Geometry check sheet. Reference: the model listing, model coordinates, mm. A direction names the side the tool comes from. Give positions to 0.01 mm unless a question says otherwise; leave off trailing zeros. Loops run counter-clockwise (first coordinate to the right, second up) from the corner with the lowest first, then second, coordinate; pieces in that order, holes last. Notation, with made-up numbers: (53, -40) -> (100, -40) arc R12 ccw to (100, -36) -> close; hole circle Ø10 at (22.5, 65). An arc over 180 degrees is marked (long way). Write item = value, one per line. Start each with the question number.
```python
from build123d import *

# Parameters (mm, degrees)
F0_W     = 600
F0_H     = 600
F1_DEPTH = 50
F2_W     = 600
F2_H     = 30
F3_DEPTH = 800
F5_DEPTH = 600


with BuildPart() as f1:
    # F0 (on Top) → F1 (new body)
    with BuildSketch(Plane.XY):
        Rectangle(F0_W, F0_H)
    extrude(amount=F1_DEPTH)

    # F2 (on face) → F3 (join)
    with BuildSketch(Plane.XY.offset(50)):
        with Locations((0, -285)):
            Rectangle(F2_W, F2_H)
    extrude(amount=F3_DEPTH)

    # F4 (on face) → F5 (join)
    with BuildSketch(Plane(origin=(0, 0, 0), x_dir=(1, 0, 0), z_dir=(0, 0, -1))):
        with BuildLine():
            Line((-250, 250), (-200, 250))
            ThreePointArc((-200, 250), (-214.644661, 285.355339), (-250, 300))
            ThreePointArc((-250, 300), (-285.355339, 285.355339), (-300, 250))
            ThreePointArc((-300, 250), (-285.355339, 214.644661), (-250, 200))
            Line((-250, 200), (-250, 250))
        make_face()
        with BuildLine():
            ThreePointArc((-250, 200), (-214.644661, 214.644661), (-200, 250))
            Line((-200, 250), (-250, 250))
            Line((-250, 250), (-250, 200))
        make_face()
        with BuildLine():
            ThreePointArc((250, 300), (214.644661, 285.355339), (200, 250))
            Line((200, 250), (250, 250))
            Line((250, 250), (250, 200))
            ThreePointArc((250, 200), (285.355339, 214.644661), (300, 250))
            ThreePointArc((300, 250), (285.355339, 285.355339), (250, 300))
        make_face()
        with BuildLine():
            ThreePointArc((-200, -250), (-214.644661, -214.644661), (-250, -200))
            Line((-250, -200), (-250, -250))
            Line((-250, -250), (-200, -250))
        make_face()
        with BuildLine():
            Line((-250, -250), (-250, -200))
            ThreePointArc((-250, -200), (-285.355339, -214.644661), (-300, -250))
            ThreePointArc((-300, -250), (-285.355339, -285.355339), (-250, -300))
            ThreePointArc((-250, -300), (-214.644661, -285.355339), (-200, -250))
            Line((-200, -250), (-250, -250))
        make_face()
        with BuildLine():
            Line((250, -250), (250, -200))
            ThreePointArc((250, -200), (214.644661, -214.644661), (200, -250))
            Line((200, -250), (250, -250))
        make_face()
        with BuildLine():
            ThreePointArc((300, -250), (285.355339, -214.644661), (250, -200))
            Line((250, -200), (250, -250))
            Line((250, -250), (200, -250))
            ThreePointArc((200, -250), (214.644661, -285.355339), (250, -300))
            ThreePointArc((250, -300), (285.355339, -285.355339), (300, -250))
        make_face()
        with BuildLine():
            Line((250, 250), (200, 250))
            ThreePointArc((200, 250), (214.644661, 214.644661), (250, 200))
            Line((250, 200), (250, 250))
        make_face()
    extrude(amount=F5_DEPTH)


solid = f1.part
```
1) Section check D-D (z = 762.5). Enter the section's corners in (x, y).
2) Draft check along X on faces 4 (the flat face through (290, -290, 0)), 5 (the flat face through (300, -90, 45)), 6 (the flat face through (-4, 4, 0)). Enter one of: released by +X, released by -X, zero draft, split by the parting line, or undercut.
3) Depth check by flat-ended pin: pin 1 Ø8 at (x, y) = (60.5, -204) entering from +Z. Enter the tip coordinate at first touch or a pass-through.
4) Section check A-A (z = -100.5). Enter the section's corners in (x, y), plus the area to 3 significant figures.
5) Section check B-B (x = 56). Enter the section's corners in (y, z), plus the area to 3 significant figures.
6) Tool access check on faces 1 (the flat face through (-290, 288, 0)), 2 (the flat face through (-290, -288, 0)), 3 (the flat face through (-4, -270, 444)). Record the directions out of +Z, -Z, +X, -X, +Y, -Y that give a thin tool (end or side, any length) a straight path to the whole face; none if there is none.
7) Thickness scan on line 1 (Z direction, x = 97, y = -217); line 2 (Z direction, x = -224, y = -217); line 3 (Y direction, x = -244, z = 522). Record the ranges inside material, lowest first.
8) Section check C-C (y = 215.5). Enter the section's corners in (x, z).
Check result:
q1.outline = (-300, -300) -> (300, -300) -> (300, -270) -> (-300, -270) -> close
q2.face_4 = zero draft
q2.face_5 = released by +X
q2.face_6 = undercut
q3.pin_1 = 50
q4.outline = circle Ø100 at (-250, -250); circle Ø100 at (-250, 250); circle Ø100 at (250, -250); circle Ø100 at (250, 250)
q4.area = 31,400 mm2
q5.outline = (-300, 0) -> (300, 0) -> (300, 50) -> (-270, 50) -> (-270, 850) -> (-300, 850) -> close
q5.area = 54,000 mm2
q6.face_1 = -Z, -X, +Y
q6.face_2 = -Z, -X, -Y
q6.face_3 = +Z, +X, -X, +Y
q7.line_1 = 0 to 50
q7.line_2 = -600 to 50
q7.line_3 = -300 to -270
q8.outline = (-300, 0) -> (-286.19, 0) -> (-286.19, -600) -> (-213.81, -600) -> (-213.81, 0) -> (213.81, 0) -> (213.81, -600) -> (286.19, -600) -> (286.19, 0) -> (300, 0) -> (300, 50) -> (-300, 50) -> close
